Read the model definition and answer for the solid it produces. Units are mm, in the model's axes. Face numbers are marked on the shaded views. Round coordinates to 2 decimals unless told otherwise and drop trailing zeros. Write each loop counter-clockwise with the first axis right and the second up, starting at its lowest first coordinate (ties: lowest second). Pieces come first, ordered by that corner, then holes.
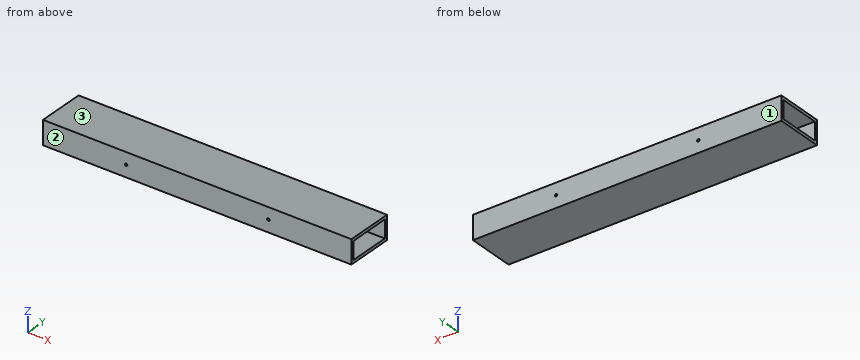
from build123d import *

# Parameters (mm, degrees)
SKETCH1_W             = 25.4
SKETCH1_H             = 50.8
SKETCH1_W_2           = 19.05
SKETCH1_H_2           = 44.45
BOSS_EXTRUDE1_DEPTH   = 330.2
F_6_32_TAPPED_HOLE6_D = 2.7051


with BuildPart() as part:
    # Sketch1 → Boss-Extrude1 (new body)
    with BuildSketch(Plane(origin=(0, 0, 0), x_dir=(0, 0, -1), z_dir=(1, 0, 0))):
        Rectangle(SKETCH1_W, SKETCH1_H)
        Rectangle(SKETCH1_W_2, SKETCH1_H_2, mode=Mode.SUBTRACT)
    extrude(amount=BOSS_EXTRUDE1_DEPTH)

    # #6-32 Tapped Hole6 (through all)
    with Locations(Plane(origin=(88.9, -25.4, 0), x_dir=(0, 0, -1), z_dir=(0, -1, 0))):
        with Locations((0, 0), (0, 152.4)):
            Hole(F_6_32_TAPPED_HOLE6_D / 2)


solid = part.part
Q1. Section B-B (x = 130) is taken. Determine the outline of the cut face in (y, z) (3 decimals), then the cut area to 3 significant figures.
Verdict:
outline: (-25.4, -12.7) - (25.4, -12.7) - (25.4, 12.7) - (-25.4, 12.7) - close; hole (-22.225, -9.525) - (22.225, -9.525) - (22.225, 9.525) - (-22.225, 9.525) - close
area: 444 mm2
Q2. A flat-ended cylindrical pin translates along its axis: pin 1 Ø1.6 at (x, z) = (241.3, 0) entering from -Y. Find the tip coordinate at first contact, or state that the pin passes through.
Verdict:
pin 1: passes through
Q3. Section A-A (y = 12.5) is taken. Determine the outline of the cut face in (x, z) (3 decimals).
Verdict:
outline: (0, -12.7) - (330.2, -12.7) - (330.2, -9.525) - (0, -9.525) - close; (0, 9.525) - (330.2, 9.525) - (330.2, 12.7) - (0, 12.7) - close
Q4. Determine the mould class of the marked faces 1, 2 and 3 for opening direction Y: pulls with the +Y half, pulls with the -Y half, needs draft (parallel to the pull), parting line crosses it, or undercut.
Verdict:
face 1: pulls with the +Y half
face 2: pulls with the -Y half
face 3: needs draft
Q5. Straight lines are drawn through the part: probe 1 along X at (y, z) = (-23.3, 0); probe 2 along Y at (x, z) = (20, -7) (3 decimals); probe 3 along Z at (x, y) = (266, -4) (3 decimals). For each, find the intervals that lie inside material, in ascending order.
Verdict:
probe 1: x = 0 to 87.55, 90.25 to 239.95, 242.65 to 330.2
probe 2: y = -25.4 to -22.225, 22.225 to 25.4
probe 3: z = -12.7 to -9.525, 9.525 to 12.7
Q6. Section C-C (z = 6) is taken. Determine the outline of the cut face in (x, y) (3 decimals).
Verdict:
outline: (0, -25.4) - (330.2, -25.4) - (330.2, -22.225) - (0, -22.225) - close; (0, 22.225) - (330.2, 22.225) - (330.2, 25.4) - (0, 25.4) - close
